Verification items for the finished model (mm, model axes). Face numbers are marked on the shaded views. A direction names the side the tool comes from. Coordinates: 2 decimals unless noted, no trailing zeros. Order: outer loops, then holes, each group sorted by start corner. A loop starts at its lowest first (then second) coordinate and runs counter-clockwise, first axis right, second up. Notation, with made-up numbers: M 4.5,16.5 L 55.5,16.5 A27 cw 55.5,54.5 Z; hole C 13,24.25 d3. An arc over 180 degrees is marked long. Answer as a JSON object with one key per item and string values. Group by question number.
(1) Cross-section at B-B (x = 50.8). Enter the section's corners in (y, z) (1 decimal).
(2) Mould release check, pull along Y, two halves, no side actions. Record for the marked faces 1, 2 and 3: released by +Y, released by -Y, zero draft, split by the parting line, or undercut.
(3) Gauge pin test, flat ends, axial feed: pin 1 Ø2 at (x, y) = (45.5, 55.5) entering from +Z; pin 2 Ø2 at (x, y) = (89.5, 104) entering from +Z. Record the tip position at first contact, or that the pin passes through.
(4) Material ranges on line 1 (Y direction, x = 11.5, z = 29.5); line 2 (Z direction, x = 76.2, y = 148) (1 decimal); line 3 (Z direction, x = 63.5, y = 24), recorded low to high.
(5) Access from +Z, -Z, +X, -X, +Y, -Y to the whole of each face (thin tool, end or side, straight path). Record for the marked faces 4 and 5.
(6) Cross-section at A-A (z = 29). Enter the section's corners in (x, y).
(7) Cross-section at C-C (z = 66.5). Enter the section's corners in (x, y), plus the area to 3 significant figures.
(8) Cross-section at D-D (z = 39). Enter the section's corners in (x, y), plus the area to 3 significant figures.
from build123d import *

# Parameters (mm, degrees)
F0_W      = 101.6
F0_H      = 148.59
F1_DEPTH  = 1.5875
F2_W      = 101.6
F2_H      = 1.5875
F3_DEPTH  = 88.9
F5_R      = 1.905
F6_DEPTH  = 1.5875
F7_R      = 1.5875
F8_DEPTH  = 1.5875
F9_W      = 6.35
F9_H      = 15.24
F10_DEPTH = 1.5875


with BuildPart() as f1:
    # F0 (on Top) → F1 (new body)
    with BuildSketch(Plane.XY):
        with Locations((50.8, 74.295)):
            Rectangle(F0_W, F0_H)
    extrude(amount=F1_DEPTH)

    # F2 (on face) → F3 (join)
    with BuildSketch(Plane.XY.offset(1.5875)):
        with Locations((50.8, 147.79625)):
            Rectangle(F2_W, F2_H)
        with Locations((50.8, 0.79375)):
            Rectangle(F2_W, F2_H)
    extrude(amount=F3_DEPTH)

    # F5 (on face) → F6 (cut, through all)
    with BuildSketch(Plane(origin=(0, 148.59, 0), x_dir=(-1, 0, 0), z_dir=(0, 1, 0))):
        with BuildLine():
            ThreePointArc((-68.58, 50.8), (-50.8, 33.02), (-33.02, 50.8))
            ThreePointArc((-33.02, 50.8), (-50.8, 68.58), (-68.58, 50.8))
        make_face()
        with BuildLine():
            ThreePointArc((-68.58, 50.8), (-50.8, 68.58), (-33.02, 50.8))
            Line((-33.02, 50.8), (-33.02, 90.4875))
            Line((-33.02, 90.4875), (-68.58, 90.4875))
            Line((-68.58, 90.4875), (-68.58, 50.8))
        make_face()
        with Locations((-50.8, 25.4)):
            Circle(F5_R)
        with Locations((-25.4, 50.8)):
            Circle(F5_R)
        with Locations((-76.2, 50.8)):
            Circle(F5_R)
    extrude(amount=-F6_DEPTH, mode=Mode.SUBTRACT)

    # F7 (on face) → F8 (cut, through all)
    with BuildSketch(Plane.XZ):
        with BuildLine():
            ThreePointArc((43.18, 50.8), (50.8, 43.18), (58.42, 50.8))
            ThreePointArc((58.42, 50.8), (50.8, 58.42), (43.18, 50.8))
        make_face()
        with BuildLine():
            ThreePointArc((43.18, 50.8), (50.8, 58.42), (58.42, 50.8))
            Line((58.42, 50.8), (58.42, 90.4875))
            Line((58.42, 90.4875), (43.18, 90.4875))
            Line((43.18, 90.4875), (43.18, 50.8))
        make_face()
        with Locations((73.9775, 50.8)):
            Circle(F7_R)
        with Locations((27.6225, 50.8)):
            Circle(F7_R)
    extrude(amount=-F8_DEPTH, mode=Mode.SUBTRACT)

    # F9 (on face) → F10 (cut, through all)
    with BuildSketch(Plane.XY.offset(1.5875)):
        with BuildLine():
            ThreePointArc((46.99, 138.7475), (43.815, 141.9225), (40.64, 138.7475))
            Line((40.64, 138.7475), (46.99, 138.7475))
        make_face()
        with Locations((43.815, 131.1275)):
            Rectangle(F9_W, F9_H)
        with BuildLine():
            Line((46.99, 123.5075), (40.64, 123.5075))
            ThreePointArc((40.64, 123.5075), (43.815, 120.3325), (46.99, 123.5075))
        make_face()
        with Locations((57.785, 131.1275)):
            Rectangle(F9_W, F9_H)
        with BuildLine():
            Line((54.61, 138.7475), (60.96, 138.7475))
            ThreePointArc((60.96, 138.7475), (57.785, 141.9225), (54.61, 138.7475))
        make_face()
        with BuildLine():
            ThreePointArc((54.61, 123.5075), (57.785, 120.3325), (60.96, 123.5075))
            Line((60.96, 123.5075), (54.61, 123.5075))
        make_face()
        with BuildLine():
            ThreePointArc((54.61, 43.4975), (57.785, 40.3225), (60.96, 43.4975))
            Line((60.96, 43.4975), (54.61, 43.4975))
        make_face()
        with Locations((57.785, 51.1175)):
            Rectangle(F9_W, F9_H)
        with BuildLine():
            Line((54.61, 58.7375), (60.96, 58.7375))
            ThreePointArc((60.96, 58.7375), (57.785, 61.9125), (54.61, 58.7375))
        make_face()
        with BuildLine():
            Line((46.99, 43.4975), (40.64, 43.4975))
            ThreePointArc((40.64, 43.4975), (43.815, 40.3225), (46.99, 43.4975))
        make_face()
        with Locations((43.815, 51.1175)):
            Rectangle(F9_W, F9_H)
        with BuildLine():
            ThreePointArc((46.99, 58.7375), (43.815, 61.9125), (40.64, 58.7375))
            Line((40.64, 58.7375), (46.99, 58.7375))
        make_face()
    extrude(amount=-F10_DEPTH, mode=Mode.SUBTRACT)


solid = f1.part
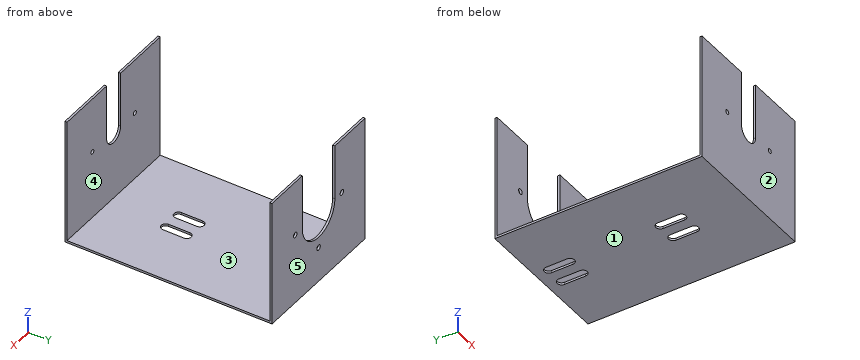
Taken from the geometry:
{
 "1": {"outline": "M 0,0 L 148.6,0 L 148.6,23.5 L 147,23.5 L 147,1.6 L 1.6,1.6 L 1.6,43.2 L 0,43.2 Z; M 147,27.3 L 148.6,27.3 L 148.6,33 L 147,33 Z"},
 "2": {"face 1": "zero draft", "face 2": "released by -Y", "face 3": "undercut"},
 "3": {"pin 1": "passes through", "pin 2": "stops at z = 1.59"},
 "4": {"line 1": "y = 0 to 1.59, 147 to 148.59", "line 2": "z = 0 to 48.9, 52.7 to 90.5", "line 3": "z = 0 to 1.59"},
 "5": {"face 4": "+Z, +X, -X", "face 5": "+Z, -Z, +X, -X, +Y"},
 "6": {"outline": "M 0,0 L 101.6,0 L 101.6,1.59 L 0,1.59 Z; M 0,147 L 101.6,147 L 101.6,148.59 L 0,148.59 Z"},
 "7": {"outline": "M 0,0 L 43.18,0 L 43.18,1.59 L 0,1.59 Z; M 0,147 L 33.02,147 L 33.02,148.59 L 0,148.59 Z; M 58.42,0 L 101.6,0 L 101.6,1.59 L 58.42,1.59 Z; M 68.58,147 L 101.6,147 L 101.6,148.59 L 68.58,148.59 Z", "area": "242 mm²"},
 "8": {"outline": "M 0,0 L 101.6,0 L 101.6,1.59 L 0,1.59 Z; M 0,147 L 37.5,147 L 37.5,148.59 L 0,148.59 Z; M 64.1,147 L 101.6,147 L 101.6,148.59 L 64.1,148.59 Z", "area": "280 mm²"}
}
